Answer from the drawing. Dimensions are ordinates in mm from the lowest x, y and z of the part. A direction names the side the tool comes from. Give positions to 0.01 mm unless a question says otherwise; leave off trailing zeros. Loops run counter-clockwise (first coordinate to the right, second up) from the corner with the lowest first, then second, coordinate; pieces in that order, holes last. Notation, with made-up numbers: (10.25, -35.75) -> (24.25, -35.75) arc R27 cw to (24.25, 3.25) -> close; hole circle Ø2 at (75, 15). An arc over 180 degrees is marked (long way). Write each question's results on one line, items separated by ' | '. Start each with the question number.
Item 1: Section B-B on x = 7.3 is taken. Write down the section's boundary in (y, z) (3 decimals), and give its area (3 significant figures).
Item 2: Find the intervals of material crossed by line 1 (X direction, y = 33.5, z = 4.75); line 2 (X direction, y = 25.5, z = 6); line 3 (Z direction, x = 11.5, y = 11.5), in increasing order.
Item 3: Each of these flat-tipped pins is pushed along its axis until it touches: P1, Ø1.3, axis at x = 7, z = 15.5, coming from the +Y side; P2, Ø3, axis at y = 12.5, z = 15.5, coming from the +X side; P3, Ø0.8, axis at y = 6, z = 15.5, coming from the -X side. Where does it stop, or does it pass through?
Item 4: Which of the six approach directions +Z, -Z, +X, -X, +Y, -Y give full straight-line access (tool end or side, diameter ignored) to the marked faces 1 and 2?
Item 5: Section D-D on y = 37 is taken. Write down the section's boundary in (x, z) (1 decimal), and give its area (3 significant figures).
Item 6: Section C-C on z = 15.5 is taken. Write down the section's boundary in (x, y).
Item 7: Section A-A on y = 16.5 is taken. Write down the section's boundary in (x, z) (1 decimal).
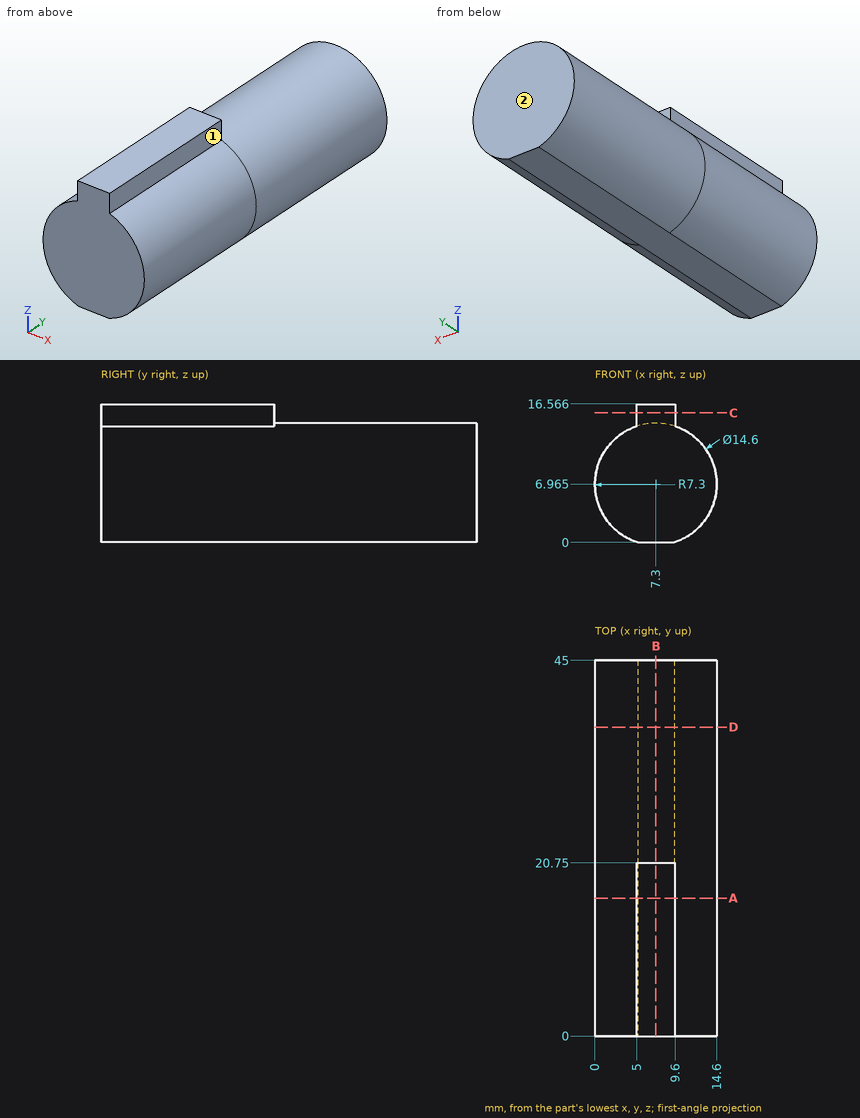
Findings:
1) outline: (0, 0) -> (45, 0) -> (45, 14.265) -> (20.75, 14.265) -> (20.75, 16.566) -> (0, 16.566) -> close | area: 690 mm2
2) line 1: 0.34 to 14.26 | line 2: 0.06 to 14.54 | line 3: 0.99 to 12.94
3) P1: y = 20.75 | P2: x = 9.6 | P3: x = 5
4) face 1: +Z, +X, +Y, -Y | face 2: +Z, -Z, +X, -X, +Y
5) outline: (5.1, 0) -> (9.5, 0) arc R7.3 ccw (long way) to start | area: 166 mm2
6) outline: (5, 0) -> (9.6, 0) -> (9.6, 20.75) -> (5, 20.75) -> close
7) outline: (5, 13.9) arc R7.3 ccw to (5.1, 0) -> (9.5, 0) arc R7.3 ccw to (9.6, 13.9) -> (9.6, 16.6) -> (5, 16.6) -> close
